from build123d import *

# Parameters (mm, degrees)
EXTRUDE_1_DEPTH     = 4
CUT_EXTRUDE_1_DEPTH = 1.5
CUT_EXTRUDE_2_DEPTH = 7.5


with BuildPart() as part:
    # Эскиз1 → Бобышка-Вытянуть1 (new body, symmetric)
    with BuildSketch(Plane.XY):
        Polygon((4, 0), (-4, 0), (-4, -1.5), (-9.75, -1.5), (-9.75, -8), (9.75, -8), (9.75, -1.5), (4, -1.5), align=None)
    extrude(amount=EXTRUDE_1_DEPTH, both=True)

    # Эскиз3 → Отверстие обработанное метчиком M43 (revolve, cut)
    with BuildSketch(Plane(origin=(0, 0, 0), x_dir=(0, 0, 1), z_dir=(1, 0, 0))):
        Polygon((0, 0), (0, 8), (2.15, 8), (1.65, 7.5), (1.65, 0.5), (2.15, 0), align=None)
    revolve(axis=Axis((0, 6.35, 0), (0, -1, 0)), mode=Mode.SUBTRACT)

    # Эскиз4 → Вырез-Вытянуть1 (cut)
    with BuildSketch(Plane(origin=(0, 0, 0), x_dir=(1, 0, 0), z_dir=(0, 1, 0))):
        with BuildLine():
            Line((-4, 4), (-4, 0))
            ThreePointArc((-4, 0), (-2.828427125, 2.828427125), (0, 4))
            Line((0, 4), (-4, 4))
        make_face()
        with BuildLine():
            Line((0, -4), (4, -4))
            Line((4, -4), (4, 0))
            ThreePointArc((4, 0), (2.828427125, -2.828427125), (0, -4))
        make_face()
    extrude(amount=-CUT_EXTRUDE_1_DEPTH, mode=Mode.SUBTRACT)

    # Эскиз5 → Вырез-Вытянуть2 (cut, through all)
    with BuildSketch(Plane(origin=(0, -1.5, 0), x_dir=(1, 0, 0), z_dir=(0, 1, 0))):
        with BuildLine():
            Line((-9.75, 0), (-9.75, 4))
            Line((-9.75, 4), (-8.891709622, 4))
            ThreePointArc((-8.891709622, 4), (-9.533012871, 2.045523305), (-9.75, 0))
        make_face()
        with BuildLine():
            Line((9.75, 0), (9.75, -4))
            Line((9.75, -4), (8.891709622, -4))
            ThreePointArc((8.891709622, -4), (9.533012871, -2.045523305), (9.75, 0))
        make_face()
    extrude(amount=-CUT_EXTRUDE_2_DEPTH, mode=Mode.SUBTRACT)

    # Вырез-По траектории1: sweep along a path in Эскиз7
    with BuildLine(Plane.XZ.offset(8)) as sweep_1_path:
        Line((0, 9.75), (-9.75, 9.75))
        Line((-9.75, 9.75), (-9.75, 0))
        ThreePointArc((-9.75, 0), (-6.894291117, -6.894291117), (0, -9.75))
        Line((0, -9.75), (9.75, -9.75))
        Line((9.75, -9.75), (9.75, 0))
        ThreePointArc((9.75, 0), (6.894291117, 6.894291117), (0, 9.75))
    # Эскиз6 → Вырез-По траектории1 (sweep, cut)
    with BuildSketch(Plane.XY.offset(4)):
        Polygon((-9.75, -3), (-9.75, -8), (-4, -8), align=None)
    sweep(path=sweep_1_path.line, transition=Transition.RIGHT, mode=Mode.SUBTRACT)


solid = part.part
Geometry: final body of the model. Coordinates: model frame, mm. A direction names the side the tool comes from. Round coordinates to 2 decimals unless told otherwise and drop trailing zeros. Loops run counter-clockwise (first coordinate to the right, second up) from the corner with the lowest first, then second, coordinate; pieces in that order, holes last.
Q1. Section A-A on y = -1.25. Return loops of the section in (x, z), plus the area to 3 significant figures.
Q2. Material intervals for L1, parallel to X at y = -2.25, z = 0; L2, parallel to Z at x = 0, y = -4.5, sorted ascending.
Q3. Section B-B on y = -2.5. Return loops of the section in (x, z), plus the area to 3 significant figures.
Q4. Access query for faces 1 (the cylindrical face through (9.527, -2.24, 2.074)), 2 (the flat face through (4, -1, -2)), 3 (the flat face through (-4, -1, 2)). Directions: +Z, -Z, +X, -X, +Y, -Y. A direction counts if a zero-diameter tool reaches every point of the face in a straight line with its end or side. Return the directions, or none.
Q5. Pin query (flat end, axial travel): P1, Ø4, axis at x = 0, z = 0, coming from the +Y side; P2, Ø0.8, axis at y = -1, z = -3, coming from the +X side; P3, Ø4, axis at y = -4, z = -2.5, coming from the -X side. Return the tip coordinate at first contact, or that it passes through.
Q6. Pull-direction query (Z, two-part tool) for faces 4 (the cylindrical face through (-1.115, -3.951, -1.216)), 5 (the cylindrical face through (-2.859, -0.74, -2.797)), 6 (the flat face through (6.835, -5.535, -1.972)); classes: released by +Z, released by -Z, zero draft, split by the parting line, or undercut.
Evaluation:
1. outline: (-4, 0) arc R4 ccw to (0, -4) - (4, -4) - (4, 0) arc R4 ccw to (0, 4) - (-4, 4) - close; hole circle Ø3.3 at (0, 0)
1. area: 48.6 mm2
2. L1: x = -9.75 to -1.65, 1.65 to 9.75
2. L2: z = -4 to -1.65, 1.65 to 4
3. outline: (-9.75, 0) arc R9.75 ccw to (-8.89, -4) - (9.75, -4) - (9.75, 0) arc R9.75 ccw to (8.89, 4) - (-9.75, 4) - close; hole circle Ø3.3 at (0, 0)
3. area: 145 mm2
4. face 1: +Z, +X, +Y, -Y
4. face 2: +Z, -Z, +X, +Y
4. face 3: +Z, -Z, -X, +Y
5. P1: stops at y = -0.15
5. P2: stops at x = 4
5. P3: stops at x = -9.72
6. face 4: undercut
6. face 5: released by -Z
6. face 6: zero draft
